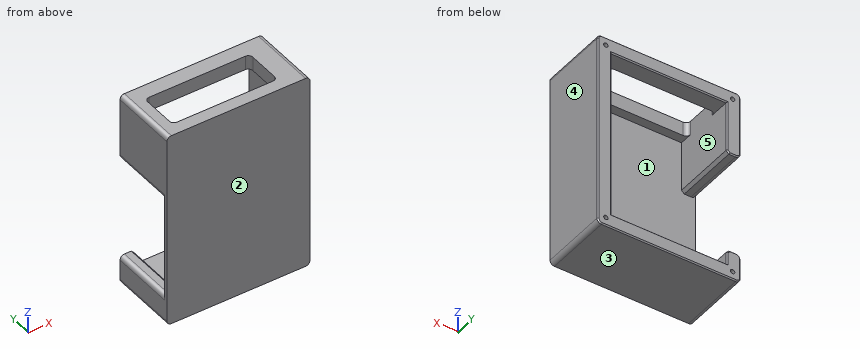
```python
from build123d import *

# Parameters (mm, degrees)
SKETCH1_W                 = 81.750000004
SKETCH1_H                 = 112.500000004
BOSS_EXTRUDE3_DEPTH       = 39.5
SHELL1_T                  = -8.000000002
SHELL1_THICKNESS_2_FACE_W = 96.5
SHELL1_THICKNESS_2_FACE_H = 65.75
SHELL1_THICKNESS_2_DEPTH  = 6.000000002
CUT_EXTRUDE1_REACH        = 149.903
SKETCH2_W                 = 58
SKETCH2_H                 = 37.5
CUT_EXTRUDE2_REACH        = 160.928
SKETCH3_W                 = 60
SKETCH3_H                 = 23
FILLET1_R                 = 2.54
CHAMFER1_SIZE             = 1.5875
FILLET2_R                 = 2.54
CHAMFER2_SIZE             = 0.635
SKETCH4_R                 = 1.25
CUT_EXTRUDE3_DEPTH        = 6.35


with BuildPart() as part:
    # Sketch1 → Boss-Extrude3 (new body)
    with BuildSketch(Plane(origin=(0, 0, 0), x_dir=(1, 0, 0), z_dir=(0, 1, 0))):
        with Locations((64.204457377, 60.506337211)):
            Rectangle(SKETCH1_W, SKETCH1_H)
    extrude(amount=BOSS_EXTRUDE3_DEPTH)

    # Shell1
    shell1_openings = [part.faces().sort_by_distance(p)[0] for p in [
        (64.204457377, 39.5, -60.506337211),
    ]]
    offset(amount=SHELL1_T, openings=shell1_openings, kind=Kind.INTERSECTION)

    # Shell1 thickness 2 face (on inner face of the shell) → Shell1 thickness 2 (cut)
    with BuildSketch(Plane(origin=(64.204457377, 8.000000002, -60.506337211), x_dir=(0, 0, -1), z_dir=(0, -1, 0))):
        Rectangle(SHELL1_THICKNESS_2_FACE_W, SHELL1_THICKNESS_2_FACE_H)
    extrude(amount=SHELL1_THICKNESS_2_DEPTH, mode=Mode.SUBTRACT)

    # Sketch2 → Cut-Extrude1 (cut, up to next)
    with BuildSketch(Plane.ZY.offset(-23.329457375), mode=Mode.PRIVATE) as cut_extrude1_sk1:
        with Locations((-71.256337211, 20.75)):
            Rectangle(SKETCH2_W, SKETCH2_H)
    cut_extrude1_tool1 = extrude(cut_extrude1_sk1.sketch, amount=-CUT_EXTRUDE1_REACH, mode=Mode.PRIVATE) & part.part
    add(cut_extrude1_tool1.solids().sort_by_distance((23.329457, 20.75, -71.256337))[0], mode=Mode.SUBTRACT)

    # Sketch3 → Cut-Extrude2 (cut, up to next)
    with BuildSketch(Plane.XY.offset(-4.256337209), mode=Mode.PRIVATE) as cut_extrude2_sk1:
        with Locations((61.329457377, 18.5)):
            Rectangle(SKETCH3_W, SKETCH3_H)
    cut_extrude2_tool1 = extrude(cut_extrude2_sk1.sketch, amount=-CUT_EXTRUDE2_REACH, mode=Mode.PRIVATE) & part.part
    add(cut_extrude2_tool1.solids().sort_by_distance((61.329457, 18.5, -4.256337))[0], mode=Mode.SUBTRACT)

    # Fillet1
    fillet1_edges = [part.edges().sort_by_distance(p)[0] for p in [
        (23.329457375, 20.75, -100.256337211),
        (23.329457375, 20.75, -42.256337211),
        (23.329457375, 19.75, -116.756337213),
        (105.079457379, 19.75, -116.756337213),
        (105.079457379, 19.75, -4.256337209),
        (23.329457375, 19.75, -4.256337209),
    ]]
    fillet(fillet1_edges, radius=FILLET1_R)

    # Chamfer1
    chamfer1_edges = [part.edges().sort_by_distance(p)[0] for p in [
        (31.329457377, 20.75, -100.256337211),
        (31.329457377, 20.75, -42.256337211),
    ]]
    chamfer(chamfer1_edges, length=CHAMFER1_SIZE)

    # Fillet2
    fillet2_edges = [part.edges().sort_by_distance(p)[0] for p in [
        (31.329457377, 7, -8.25633721),
        (31.329457377, 30, -8.25633721),
        (91.329457377, 30, -8.25633721),
        (91.329457377, 7, -8.25633721),
    ]]
    fillet(fillet2_edges, radius=FILLET2_R)

    # Chamfer2
    chamfer2_edges = [part.edges().sort_by_distance(p)[0] for p in [
        (31.329457377, 39.5, -26.462587211),
        (27.805707376, 39.5, -42.256337211),
        (27.805707376, 39.5, -100.256337211),
        (30.535707377, 39.5, -101.050087211),
        (30.535707377, 39.5, -41.462587211),
        (31.329457377, 39.5, -105.300087211),
        (64.204457377, 39.5, -12.256337211),
        (97.079457377, 39.5, -60.506337211),
        (64.204457377, 39.5, -108.756337211),
        (23.329457375, 39.5, -23.25633721),
        (64.204457377, 39.5, -4.256337209),
        (105.079457379, 39.5, -60.506337211),
        (64.204457377, 39.5, -116.756337213),
        (23.329457375, 39.5, -108.506337212),
        (104.335508603, 39.5, -116.012388437),
        (104.335508603, 39.5, -5.000285984),
        (24.073406151, 39.5, -5.000285984),
        (24.073406151, 39.5, -116.012388437),
        (24.073406151, 39.5, -101.000285986),
        (24.073406151, 39.5, -41.512388435),
    ]]
    chamfer(chamfer2_edges, length=CHAMFER2_SIZE)

    # Sketch4 → Cut-Extrude3 (cut)
    with BuildSketch(Plane(origin=(0, 39.5, 0), x_dir=(1, 0, 0), z_dir=(0, 1, 0))):
        with Locations(Location((27.964457375, 112.121337213, 0), (0, 0, 270))):
            Circle(SKETCH4_R)
        with Locations(Location((100.444457379, 112.121337213, 0), (0, 0, 270))):
            Circle(SKETCH4_R)
        with Locations(Location((27.964457375, 8.891337209, 0), (0, 0, 270))):
            Circle(SKETCH4_R)
        with Locations(Location((100.444457379, 8.891337209, 0), (0, 0, 270))):
            Circle(SKETCH4_R)
    extrude(amount=-CUT_EXTRUDE3_DEPTH, mode=Mode.SUBTRACT)


solid = part.part
```
Source: CAD feature listing. Evaluate the final solid. Frame: model axes, mm. Face numbers are marked on the shaded views. A direction names the side the tool comes from. Round coordinates to 2 decimals unless told otherwise and drop trailing zeros. Loops run counter-clockwise (first coordinate to the right, second up) from the corner with the lowest first, then second, coordinate; pieces in that order, holes last. Notation, with made-up numbers: M 48.25,28.5 L 76.25,28.5 A20 cw 76.25,39.5 Z; hole C -23.5,68.25 d2. An arc over 180 degrees is marked long. Use a Markdown table: item, result. Add a question column.
1. Section query B-B on y = 20. Return the cut outline in (x, z).
2. Reachability of the marked faces 1 and 2 from +Z, -Z, +X, -X, +Y, -Y: full face, straight path, thin tool, end or side. Return the list, or none.
3. Section query A-A on x = 87.5. Return the cut outline in (y, z) (3 decimals).
4. Contact query for flat-ended pins moving along their axis: P1, Ø0.8, axis at x = 28, z = -8.5, coming from the +Y side; P2, Ø2, axis at x = 73.5, z = -76, coming from the -Y side; P3, Ø6, axis at y = 10, z = -68, coming from the -X side; P4, Ø1.5, axis at x = 44.5, y = 28.5, coming from the +Z side. Output: stop coordinate, or through.
5. Line query: line 1 (X direction, y = 11, z = -9.5); line 2 (X direction, y = 34, z = -15.5); line 3 (Z direction, x = 71.5, y = 32). Output: solid intervals per line, ascending.
6. Mould query, pull axis Z, two halves, no side actions, for the marked faces 3, 4 and 5. Classes: pulls with the +Z half, pulls with the -Z half, needs draft (parallel to the pull), parting line crosses it, or undercut.
7. Section query C-C on z = -32.5. Return the cut outline in (x, y) (3 decimals), then the cut area to 3 significant figures.
8. Section query D-D on y = 4. Return the cut outline in (x, z), then the cut area to 3 significant figures.
Reported:
| question | item | result |
|---|---|---|
| 1 | outline | M 23.33,-114.22 A2.54 ccw 25.87,-116.76 L 102.54,-116.76 A2.54 ccw 105.08,-114.22 L 105.08,-6.8 A2.54 ccw 102.54,-4.26 L 91.33,-4.26 L 91.33,-12.26 L 97.08,-12.26 L 97.08,-108.76 L 31.33,-108.76 L 31.33,-101.84 L 29.74,-100.26 L 25.87,-100.26 A2.54 ccw 23.33,-102.8 Z; M 23.33,-39.72 A2.54 ccw 25.87,-42.26 L 29.74,-42.26 L 31.33,-40.67 L 31.33,-4.26 L 25.87,-4.26 A2.54 ccw 23.33,-6.8 Z |
| 2 | face 1 | +Y |
| 2 | face 2 | +Z, -Z, +X, -X, -Y |
| 3 | outline | M 0,-116.756 L 38.865,-116.756 L 39.5,-116.121 L 39.5,-109.391 L 38.865,-108.756 L 2,-108.756 L 2,-12.256 L 7,-12.256 L 7,-4.256 L 0,-4.256 Z; M 30,-12.256 L 38.865,-12.256 L 39.5,-11.621 L 39.5,-4.891 L 38.865,-4.256 L 30,-4.256 Z |
| 4 | P1 | stops at y = 33.15 |
| 4 | P2 | stops at y = 0 |
| 4 | P3 | stops at x = 97.08 |
| 4 | P4 | stops at z = -108.76 |
| 5 | line 1 | x = 23.33 to 31.33, 91.33 to 105.08 |
| 5 | line 2 | x = 23.33 to 31.33, 97.08 to 105.08 |
| 5 | line 3 | z = -116.76 to -108.76, -12.26 to -4.26 |
| 6 | face 3 | pulls with the -Z half |
| 6 | face 4 | needs draft |
| 6 | face 5 | undercut |
| 7 | outline | M 23.329,0 L 105.079,0 L 105.079,38.865 L 104.444,39.5 L 97.714,39.5 L 97.079,38.865 L 97.079,2 L 31.329,2 L 31.329,38.865 L 30.694,39.5 L 23.964,39.5 L 23.329,38.865 Z |
| 7 | area | 763 mm² |
| 8 | outline | M 23.33,-114.22 A2.54 ccw 25.87,-116.76 L 102.54,-116.76 A2.54 ccw 105.08,-114.22 L 105.08,-6.8 A2.54 ccw 102.54,-4.26 L 25.87,-4.26 A2.54 ccw 23.33,-6.8 L 23.33,-39.72 A2.54 ccw 25.87,-42.26 L 29.74,-42.26 L 31.33,-40.67 L 31.33,-12.26 L 97.08,-12.26 L 97.08,-108.76 L 31.33,-108.76 L 31.33,-101.84 L 29.74,-100.26 L 25.87,-100.26 A2.54 ccw 23.33,-102.8 Z |
| 8 | area | 2,380 mm² |
